Verification items for the finished model (mm, model axes). A direction names the side the tool comes from. Round coordinates to 2 decimals unless told otherwise and drop trailing zeros. Write each loop counter-clockwise with the first axis right and the second up, starting at its lowest first coordinate (ties: lowest second). Pieces come first, ordered by that corner, then holes. Notation, with made-up numbers: (-14, 59) -> (0, 59) arc R16 cw to (0, 67) -> close; hole circle Ø8 at (-25, 5.25). An arc over 180 degrees is marked (long way). Answer as a JSON object with one key per item and string values. Group by question number.
(1) Set-up check for faces 1 (the face through (-1, 1, 26)), 2 (the face through (-55.55, -42.594, 21.07)): record each of +Z, -Z, +X, -X, +Y, -Y from which the full face is reachable in a straight line by a thin tool's end or side.
(2) Sectioned sample at A-A on x = 0. Record the cut outline in (y, z).
(3) Sectioned sample at C-C on z = 18.5. Record the cut outline in (x, y), and give its area (3 significant figures).
(4) Sectioned sample at D-D on z = 4.5. Record the cut outline in (x, y).
(5) Gauge pin test, flat ends, axial feed: pin 1 Ø2 at (y, z) = (37.5, -12) entering from +X; pin 2 Ø1 at (y, z) = (62, -16.5) entering from -X; pin 3 Ø6 at (x, z) = (10, 13) entering from -Y. Record the tip position at first contact, or that the pin passes through.
(6) Scan lines: L1, parallel to Z at x = 54, y = 47.5; L2, parallel to X at y = 18, z = 14; L3, parallel to Y at x = -1.5, z = -22. Record each from-to range of solid material in increasing order. Write a range as from..to.
```python
from build123d import *

# Parameters (mm, degrees)
SKETCH1_R           = 87.5
BOSS_EXTRUDE1_DEPTH = 26
SKETCH2_R           = 107.528589123
SKETCH2_R_2         = 70
CUT_EXTRUDE1_DEPTH  = 10
CHAMFER1_SIZE       = 5
FILLET1_R           = 3


with BuildPart() as part:
    # Sketch1 → Boss-Extrude1 (new body, symmetric)
    with BuildSketch(Plane.XY):
        Circle(SKETCH1_R)
    extrude(amount=BOSS_EXTRUDE1_DEPTH, both=True)

    # Sketch2 → Cut-Extrude1 (cut)
    with BuildSketch(Plane.XY.offset(26)):
        Circle(SKETCH2_R)
        Circle(SKETCH2_R_2, mode=Mode.SUBTRACT)
    extrude(amount=-CUT_EXTRUDE1_DEPTH, mode=Mode.SUBTRACT)

    # Chamfer1
    chamfer1_edges = [part.edges().sort_by_distance(p)[0] for p in [
        (-87.5, 0, 16),
    ]]
    chamfer(chamfer1_edges, length=CHAMFER1_SIZE)

    # Fillet1
    fillet1_edges = [part.edges().sort_by_distance(p)[0] for p in [
        (-87.5, 0, -26),
    ]]
    fillet(fillet1_edges, radius=FILLET1_R)


solid = part.part
```
Computed values:
{
 "1": {"face 1": "+Z, +X, -X, +Y, -Y", "face 2": "+Z"},
 "2": {"outline": "(-87.5, -23) arc R3 ccw to (-84.5, -26) -> (84.5, -26) arc R3 ccw to (87.5, -23) -> (87.5, 11) -> (82.5, 16) -> (70, 16) -> (70, 26) -> (-70, 26) -> (-70, 16) -> (-82.5, 16) -> (-87.5, 11) -> close"},
 "3": {"outline": "circle Ø140 at (0, 0)", "area": "15,400 mm2"},
 "4": {"outline": "circle Ø175 at (0, 0)"},
 "5": {"pin 1": "x = 79.52", "pin 2": "x = -62.24", "pin 3": "y = -87.15"},
 "6": {"L1": "-26..16", "L2": "-82.56..82.56", "L3": "-87.49..87.49"}
}
